from build123d import *

# Parameters (mm, degrees)
ESBO_O1_R                  = 5
RESSALTO_EXTRUS_O1_DEPTH   = 15
FURO_COM_FOLGA_DE_M61_D    = 6.6
CORTE_EXTRUS_O1_DEPTH      = 43.535279475
CORTE_EXTRUS_O1_DEPTH_BACK = 43.535279475
ESBO_O4_R                  = 5


with BuildPart() as part:
    # Esboço1 → Ressalto-extrusão1 (new body)
    with BuildSketch(Plane.XY):
        with BuildLine():
            Line((-5, -20), (-5, -35.5))
            Line((-5, -35.5), (5, -35.5))
            Line((5, -35.5), (5, -20))
            ThreePointArc((5, -20), (5.585786438, -18.585786438), (7, -18))
            Line((7, -18), (11, -18))
            ThreePointArc((11, -18), (15.949747468, -15.949747468), (18, -11))
            Line((18, -11), (18, 11))
            ThreePointArc((18, 11), (15.949747468, 15.949747468), (11, 18))
            Line((11, 18), (7, 18))
            ThreePointArc((7, 18), (5.585786438, 18.585786438), (5, 20))
            Line((5, 20), (5, 35.5))
            Line((5, 35.5), (-5, 35.5))
            Line((-5, 35.5), (-5, 20))
            ThreePointArc((-5, 20), (-5.585786438, 18.585786438), (-7, 18))
            Line((-7, 18), (-11, 18))
            ThreePointArc((-11, 18), (-15.949747468, 15.949747468), (-18, 11))
            Line((-18, 11), (-18, -11))
            ThreePointArc((-18, -11), (-15.949747468, -15.949747468), (-11, -18))
            Line((-11, -18), (-7, -18))
            ThreePointArc((-7, -18), (-5.585786438, -18.585786438), (-5, -20))
        make_face()
        Circle(ESBO_O1_R, mode=Mode.SUBTRACT)
    extrude(amount=RESSALTO_EXTRUS_O1_DEPTH)

    # Furo com folga de M61 (through all)
    with Locations(Plane.XY.offset(15)):
        with Locations((11, 11), (-11, 11), (-11, -11), (11, -11)):
            Hole(FURO_COM_FOLGA_DE_M61_D / 2)

    # Esboço4 → Corte-extrusão1 (cut, two sides: drawn at the far end of the back side and taken through both)
    with BuildSketch(Plane(origin=(0, 0, 0), x_dir=(0, 0, -1), z_dir=(1, 0, 0)).offset(-CORTE_EXTRUS_O1_DEPTH_BACK)):
        with Locations(Location((-7.5, 27.75, 0), (0, 0, 90))):
            Circle(ESBO_O4_R)
        with Locations(Location((-7.5, -27.75, 0), (0, 0, 90))):
            Circle(ESBO_O4_R)
    extrude(amount=CORTE_EXTRUS_O1_DEPTH + CORTE_EXTRUS_O1_DEPTH_BACK, mode=Mode.SUBTRACT)


solid = part.part
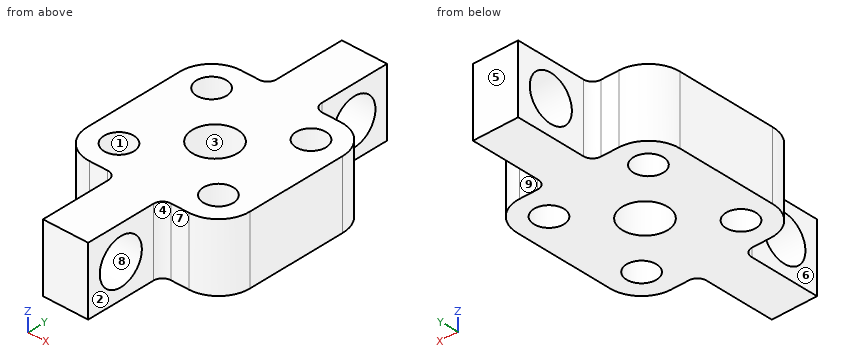
Could you check a few things on this model? Use its own coordinates, in mm. Face numbers are marked on the shaded views. A direction names the side the tool comes from. Coordinates: 2 decimals unless noted, no trailing zeros. Write each loop counter-clockwise with the first axis right and the second up, starting at its lowest first coordinate (ties: lowest second). Pieces come first, ordered by that corner, then holes. Notation, with made-up numbers: M 17.25,-2.5 L 66.25,-2.5 A30 ccw 66.25,23.5 Z; hole C -27,-39 d3. An arc over 180 degrees is marked long. One line per question, with ' | ' between items.
1) If we mould it in two halves opening along Y, with no side actions, what happens to the marked faces 1, 2, 3 and 4? For each: released by +Y, released by -Y, zero draft, split by the parting line, or undercut.
Checks:
face 1: undercut | face 2: zero draft | face 3: undercut | face 4: released by -Y
2) For pin 1 Ø2 at (x, z) = (-8.5, 5.5) entering from -Y; pin 2 Ø2 at (x, y) = (0.5, 13.5) entering from -Z; pin 3 Ø1.2 at (x, z) = (-9.5, 10) entering from +Y, each with a flat end and sliding along its axis, tell me the tip position at first contact or that it passes through.
Checks:
pin 1: y = -18 | pin 2: z = 0 | pin 3: y = 18
3) Imagine slicing it at A-A, the plane z = 4.5. Give the number of separate pieces and of enclosed holes in the cut face, and give its area (3 significant figures).
Checks:
separate pieces: 3 | enclosed holes: 5 | area: 1,230 mm²
4) I need wall thicknesses on probe 1 along Y at (x, z) = (-11, 11); probe 2 along Y at (x, z) = (0, 8); probe 3 along Y at (x, z) = (-8, 1). Which ranges of each line are inside material? Lowest first, please. Write a range as [from, to].
Checks:
probe 1: [-18, -14.3], [-7.7, 7.7], [14.3, 18] | probe 2: [-35.5, -32.72], [-22.78, -5], [5, 22.78], [32.72, 35.5] | probe 3: [-18, -12.37], [-9.63, 9.63], [12.37, 18]
5) For the marked faces 5, 6, 7, 8 and 9, which set-ups out of +Z, -Z, +X, -X, +Y, -Y let a thin tool reach every point of the face, with its end or its side?
Checks:
face 5: +Z, -Z, +X, -X, +Y | face 6: +Z, -Z, -X, -Y | face 7: +Z, -Z, +X, -Y | face 8: +X, -X | face 9: +Z, -Z, +X, +Y
6) Imagine slicing it at B-B, the plane x = -3. Write out the boundary of the cut face in (y, z).
Checks:
outline: M -35.5,0 L -4,0 L -4,15 L -35.5,15 Z; M 4,0 L 35.5,0 L 35.5,15 L 4,15 Z; hole C -27.75,7.5 d10; hole C 27.75,7.5 d10
7) Imagine slicing it at C-C, the plane z = 14. Write out the boundary of the cut face in (x, y).
Checks:
outline: M -18,-11 A7 ccw -11,-18 L -7,-18 A2 cw -5,-20 L -5,-35.5 L 5,-35.5 L 5,-20 A2 cw 7,-18 L 11,-18 A7 ccw 18,-11 L 18,11 A7 ccw 11,18 L 7,18 A2 cw 5,20 L 5,35.5 L -5,35.5 L -5,20 A2 cw -7,18 L -11,18 A7 ccw -18,11 Z; hole C -11,-11 d6.6; hole C -11,11 d6.6; hole C 0,0 d10; hole C 11,-11 d6.6; hole C 11,11 d6.6
8) Imagine slicing it at D-D, the plane y = 0. Write out the boundary of the cut face in (x, z), and give its area (3 significant figures).
Checks:
outline: M -18,0 L -5,0 L -5,15 L -18,15 Z; M 5,0 L 18,0 L 18,15 L 5,15 Z | area: 390 mm²
